Input: part model. Units: mm. Frame: model coordinates. A direction names the side the tool comes from. Give positions to 0.01 mm unless a question says otherwise; leave off trailing zeros. Loops run counter-clockwise (first coordinate to the right, second up) from the corner with the lowest first, then second, coordinate; pieces in that order, holes last.
from build123d import *

# Parameters (mm, degrees)
SKIZZE1_R                       = 28.5
AUFSATZ_LINEAR_AUSTRAGEN1_DEPTH = 43
AUFSATZ_LINEAR_AUSTRAGEN2_DEPTH = 5.2
AUFSATZ_LINEAR_AUSTRAGEN3_DEPTH = 5.3
SKIZZE4_R                       = 6.33
AUFSATZ_LINEAR_AUSTRAGEN4_DEPTH = 25
M6X1_0_GEWINDEBOHRUNG1_D        = 5
M6X1_0_GEWINDEBOHRUNG1_DEPTH    = 5.2
F_5_0_5_DURCHMESSER_BOHRUNG1_D  = 5


with BuildPart() as part:
    # Skizze1 → Aufsatz-Linear austragen1 (new body)
    with BuildSketch(Plane.XY):
        Circle(SKIZZE1_R)
    extrude(amount=AUFSATZ_LINEAR_AUSTRAGEN1_DEPTH)

    # Skizze2 → Aufsatz-Linear austragen2 (add)
    with BuildSketch(Plane.XY.offset(43)):
        Polygon((28.7, 0), (28.7, 28.7), (-28.7, 28.7), (-28.7, -28.7), (28.7, -28.7), align=None)
    extrude(amount=AUFSATZ_LINEAR_AUSTRAGEN2_DEPTH)

    # Skizze3 → Aufsatz-Linear austragen3 (add)
    with BuildSketch(Plane(origin=(0, 0, 0), x_dir=(-1, 0, 0), z_dir=(0, 0, -1))):
        Polygon((28.7, 0), (28.7, 28.7), (-28.7, 28.7), (-28.7, -28.7), (28.7, -28.7), align=None)
    extrude(amount=AUFSATZ_LINEAR_AUSTRAGEN3_DEPTH)

    # Skizze4 → Aufsatz-Linear austragen4 (add)
    with BuildSketch(Plane.XY.offset(48.2)):
        Circle(SKIZZE4_R)
    extrude(amount=AUFSATZ_LINEAR_AUSTRAGEN4_DEPTH)

    # M6x1.0 Gewindebohrung1
    with Locations(Plane.XY.offset(48.2)):
        with Locations((-23.5, 23.5), (23.5, 23.5), (23.5, -23.5), (-23.5, -23.5)):
            Hole(M6X1_0_GEWINDEBOHRUNG1_D / 2, depth=M6X1_0_GEWINDEBOHRUNG1_DEPTH)

    # Ø5.0 (5) Durchmesser Bohrung1 (through all)
    with Locations(Plane.XY.offset(48.2)):
        with Locations((-23.5, 23.5), (23.5, 23.5), (23.5, -23.5), (-23.5, -23.5)):
            Hole(F_5_0_5_DURCHMESSER_BOHRUNG1_D / 2)


solid = part.part
(1) Mould query, pull axis X, two halves, no side actions, for faces 1 (the cylindrical face through (6.04, 1.9, 60.53)), 2 (the flat face through (0, 0, -5.3)), 3 (the cylindrical face through (-21.66, 25.19, 45.56)), 4 (the flat face through (-28.7, 0, 46)). Classes: +X half, -X half, draft (parallel to the pull), parting line (faces both ways), or undercut.
Values follow:
face 1: parting line
face 2: draft
face 3: undercut
face 4: -X half
(2) Reachability of faces 5 (the cylindrical face through (25.34, 25.19, -2.69)), 6 (the cylindrical face through (26.327, -10.916, 21.199)) from +Z, -Z, +X, -X, +Y, -Y: full face, straight path, thin tool, end or side. Return the list, or none.
Values follow:
face 5: +Z, -Z
face 6: none
(3) Cut plane D-D (y = 24.5). Return the cut outline in (x, z), and give its area (3 significant figures).
Values follow:
outline: (-28.7, -5.3) - (-25.79, -5.3) - (-25.79, 0) - (-28.7, 0) - close; (-28.7, 43) - (-25.79, 43) - (-25.79, 48.2) - (-28.7, 48.2) - close; (-21.21, -5.3) - (21.21, -5.3) - (21.21, 0) - (14.56, 0) - (14.56, 43) - (21.21, 43) - (21.21, 48.2) - (-21.21, 48.2) - (-21.21, 43) - (-14.56, 43) - (-14.56, 0) - (-21.21, 0) - close; (25.79, -5.3) - (28.7, -5.3) - (28.7, 0) - (25.79, 0) - close; (25.79, 43) - (28.7, 43) - (28.7, 48.2) - (25.79, 48.2) - close
area: 1,760 mm2
(4) Cut plane A-A (x = 23.5). Return the cut outline in (y, z), and give its area (3 significant figures).
Values follow:
outline: (-28.7, -5.3) - (-26, -5.3) - (-26, 0) - (-28.7, 0) - close; (-28.7, 43) - (-26, 43) - (-26, 48.2) - (-28.7, 48.2) - close; (-21, -5.3) - (21, -5.3) - (21, 0) - (16.12, 0) - (16.12, 43) - (21, 43) - (21, 48.2) - (-21, 48.2) - (-21, 43) - (-16.12, 43) - (-16.12, 0) - (-21, 0) - close; (26, -5.3) - (28.7, -5.3) - (28.7, 0) - (26, 0) - close; (26, 43) - (28.7, 43) - (28.7, 48.2) - (26, 48.2) - close
area: 1,880 mm2
(5) Cut plane C-C (z = 45). Return the cut outline in (x, y), and give its area (3 significant figures).
Values follow:
outline: (-28.7, -28.7) - (28.7, -28.7) - (28.7, 28.7) - (-28.7, 28.7) - close; hole circle Ø5 at (-23.5, -23.5); hole circle Ø5 at (-23.5, 23.5); hole circle Ø5 at (23.5, -23.5); hole circle Ø5 at (23.5, 23.5)
area: 3,220 mm2
(6) Pin query (flat end, axial travel): pin 1 Ø2 at (x, z) = (-9, 41) entering from +Y; pin 2 Ø3 at (x, y) = (23.5, 23.5) entering from +Z; pin 3 Ø4 at (x, z) = (0.5, 52) entering from -Y; pin 4 Ø8 at (y, z) = (-17.5, 18.5) entering from -X. Return the tip coordinate at first contact, or that it passes through.
Values follow:
pin 1: stops at y = 27.35
pin 2: passes through
pin 3: stops at y = -6.33
pin 4: stops at x = -25.1
(7) Ray query, probe 1 along Y at (x, z) = (23.5, -2.85); probe 2 along Y at (x, z) = (-23, 45); probe 3 along Z at (x, y) = (20.5, 20). Return the intervals inside material, ascending.
Values follow:
probe 1: y = -28.7 to -26, -21 to 21, 26 to 28.7
probe 2: y = -28.7 to -25.95, -21.05 to 21.05, 25.95 to 28.7
probe 3: z = -5.3 to 0, 43 to 48.2
(8) Cut plane B-B (x = 0). Return the cut outline in (y, z).
Values follow:
outline: (-28.7, -5.3) - (28.7, -5.3) - (28.7, 0) - (28.5, 0) - (28.5, 43) - (28.7, 43) - (28.7, 48.2) - (6.33, 48.2) - (6.33, 73.2) - (-6.33, 73.2) - (-6.33, 48.2) - (-28.7, 48.2) - (-28.7, 43) - (-28.5, 43) - (-28.5, 0) - (-28.7, 0) - close
